```python
from build123d import *

# Parameters (mm, degrees)
SWEEP_THIN1_PROFILE_R    = 32
SWEEP_THIN1_PROFILE_R_2  = 22.5
SKETCH16_R               = 60
SKETCH16_R_2             = 7.5
SKETCH16_R_3             = 22.5
BOSS_EXTRUDE1_DEPTH      = 15
BOSS_EXTRUDE2_START      = 15
SKETCH17_R               = 60
SKETCH17_R_2             = 22.5
SKETCH17_R_3             = 7.5
BOSS_EXTRUDE2_DEPTH      = 15
SKETCH24_R               = 12
BOSS_EXTRUDE3_DEPTH      = 20
EXTRUDE_THIN1_REACH      = 577.336
EXTRUDE_THIN1_END_RADIUS = 32
SKETCH26_W               = 20
SKETCH26_H               = 64
RIB1_REACH               = 568.248
SKETCH27_WALL_W          = 1227.903575826
SKETCH27_WALL_H          = 24
SKETCH28_R               = 18
SKETCH28_R_2             = 12
BOSS_EXTRUDE4_DEPTH      = 8


with BuildPart() as part:
    # Sweep-Thin1: sweep along a path in Sketch1
    with BuildLine(Plane(origin=(0, 0, 0), x_dir=(0, 0, -1), z_dir=(1, 0, 0))) as sweep_thin1_path:
        Line((0, 0), (0, -135))
        ThreePointArc((0, -135), (-23.431457505, -191.568542495), (-80, -215))
        Line((-80, -215), (-445.82, -215))
    # Sweep-Thin1 profile (on start of the path) → Sweep-Thin1 (sweep)
    with BuildSketch(Plane(origin=(0, 0, 0), x_dir=(0, 0, -1), z_dir=(0, -1, 0))):
        Circle(SWEEP_THIN1_PROFILE_R)
        Circle(SWEEP_THIN1_PROFILE_R_2, mode=Mode.SUBTRACT)
    sweep(path=sweep_thin1_path.line)

    # Sketch16 → Boss-Extrude1 (add)
    with BuildSketch(Plane(origin=(0, 0, 0), x_dir=(1, 0, 0), z_dir=(0, 1, 0))):
        with Locations(Location((0, 0, 0), (0, 0, 270))):
            Circle(SKETCH16_R)
        with Locations(Location((0, -45, 0), (0, 0, 270))):
            Circle(SKETCH16_R_2, mode=Mode.SUBTRACT)
        with Locations(Location((-45, 0, 0), (0, 0, 270))):
            Circle(SKETCH16_R_2, mode=Mode.SUBTRACT)
        with Locations(Location((0, 45, 0), (0, 0, 270))):
            Circle(SKETCH16_R_2, mode=Mode.SUBTRACT)
        with Locations(Location((45, 0, 0), (0, 0, 270))):
            Circle(SKETCH16_R_2, mode=Mode.SUBTRACT)
        with Locations(Location((0, 0, 0), (0, 0, 90))):
            Circle(SKETCH16_R_3, mode=Mode.SUBTRACT)
    extrude(amount=BOSS_EXTRUDE1_DEPTH)

    # Sketch17 → Boss-Extrude2 (add)
    with BuildSketch(Plane.XY.offset(445.82).offset(BOSS_EXTRUDE2_START)):
        with Locations((0, -215)):
            Circle(SKETCH17_R)
        with Locations(Location((0, -215, 0), (0, 0, 270))):
            Circle(SKETCH17_R_2, mode=Mode.SUBTRACT)
        with Locations((0, -260)):
            Circle(SKETCH17_R_3, mode=Mode.SUBTRACT)
        with Locations((-45, -215)):
            Circle(SKETCH17_R_3, mode=Mode.SUBTRACT)
        with Locations((45, -215)):
            Circle(SKETCH17_R_3, mode=Mode.SUBTRACT)
        with Locations((0, -170)):
            Circle(SKETCH17_R_3, mode=Mode.SUBTRACT)
    extrude(amount=-BOSS_EXTRUDE2_DEPTH)



with BuildPart() as body_2:
    # Sketch24 → Boss-Extrude3 (new body)
    with BuildSketch(Plane(origin=(0, -325, 0), x_dir=(1, 0, 0), z_dir=(0, 1, 0))):
        with BuildLine():
            Line((15.39090645, -446.133712262), (97.89090645, -416.106167935))
            ThreePointArc((97.89090645, -416.106167935), (127.5, -373.82), (97.89090645, -331.533832065))
            Line((97.89090645, -331.533832065), (15.39090645, -301.506287738))
            ThreePointArc((15.39090645, -301.506287738), (0, -298.792455673), (-15.39090645, -301.506287738))
            Line((-15.39090645, -301.506287738), (-97.89090645, -331.533832065))
            ThreePointArc((-97.89090645, -331.533832065), (-127.5, -373.82), (-97.89090645, -416.106167935))
            Line((-97.89090645, -416.106167935), (-15.39090645, -446.133712262))
            ThreePointArc((-15.39090645, -446.133712262), (0, -448.847544327), (15.39090645, -446.133712262))
        make_face()
        with Locations(Location((-82.5, -373.82, 0), (0, 0, 270))):
            Circle(SKETCH24_R, mode=Mode.SUBTRACT)
        with Locations(Location((82.5, -373.82, 0), (0, 0, 270))):
            Circle(SKETCH24_R, mode=Mode.SUBTRACT)
    extrude(amount=BOSS_EXTRUDE3_DEPTH)


with BuildPart() as part_1:
    add(part.part)

    add(body_2.part)  # Extrude-Thin1 merges body 2
    # Extrude-Thin1: up to this cylinder (the profile starts outside it)
    extrude_thin1_end = Plane(origin=(0, -215, 373.82), z_dir=(0, 0, 1)) * Cylinder(EXTRUDE_THIN1_END_RADIUS, 1219.672, mode=Mode.PRIVATE)
    # Sketch26 → Extrude-Thin1 (add, up to the surface)
    with BuildSketch(Plane(origin=(0, -305, 0), x_dir=(1, 0, 0), z_dir=(0, 1, 0)), mode=Mode.PRIVATE) as extrude_thin1_sk1:
        with Locations((0, -373.82)):
            Rectangle(SKETCH26_W, SKETCH26_H)
    extrude_thin1_tool1 = extrude(extrude_thin1_sk1.sketch, amount=EXTRUDE_THIN1_REACH, mode=Mode.PRIVATE) - extrude_thin1_end
    add(extrude_thin1_tool1.solids().sort_by_distance((0, -305, 373.82))[0])

    # Sketch27 wall → Rib1 (add, up to next)
    with BuildSketch(Plane(origin=(44.5, -260, 385.82), x_dir=(-0.267643863786, 0.96351790963, 0), z_dir=(0.96351790963, 0.267643863786, 0)), mode=Mode.PRIVATE) as rib1_sk1:
        Rectangle(SKETCH27_WALL_W, SKETCH27_WALL_H)
    rib1_tool1 = extrude(rib1_sk1.sketch, amount=-RIB1_REACH, mode=Mode.PRIVATE) - part_1.part
    rib1 = rib1_tool1.solids().sort_by_distance((44.5, -260, 385.82))[0]
    add(rib1)

    # Mirror3: Rib1 across plane
    add(rib1.mirror(Plane(origin=(0, 0, 0), x_dir=(0, 0, 1), z_dir=(1, 0, 0))))

    # Sketch28 → Boss-Extrude4 (add)
    # profile 1 of 2: a face of its own
    with BuildSketch(Plane(origin=(0, -305, 0), x_dir=(1, 0, 0), z_dir=(0, 1, 0))):
        with Locations(Location((-82.5, -373.82, 0), (0, 0, 270))):
            Circle(SKETCH28_R)
        with Locations(Location((-82.5, -373.82, 0), (0, 0, 270))):
            Circle(SKETCH28_R_2, mode=Mode.SUBTRACT)
    # profile 2 of 2: a face of its own
    with BuildSketch(Plane(origin=(0, -305, 0), x_dir=(1, 0, 0), z_dir=(0, 1, 0))):
        with Locations(Location((82.5, -373.82, 0), (0, 0, 270))):
            Circle(SKETCH28_R)
        with Locations(Location((82.5, -373.82, 0), (0, 0, 270))):
            Circle(SKETCH28_R_2, mode=Mode.SUBTRACT)
    extrude(amount=BOSS_EXTRUDE4_DEPTH)


solid = part_1.part
```
Build history of the part. All positions in model axes, mm. A direction names the side the tool comes from. Give positions to 0.01 mm unless a question says otherwise; leave off trailing zeros. Order: outer loops, then holes, each group sorted by start corner. A loop starts at its lowest first (then second) coordinate and runs counter-clockwise, first axis right, second up. Notation, with made-up numbers: M 10,43 L 31,43 A23 cw 31,80 Z; hole C 88.5,21.25 d10. An arc over 180 degrees is marked long. Return JSON: item names as keys, results as strings.
Q1. Band-saw the part on A-A (z = 317). Give the cut face in (x, y).
Answer list:
{"outline": "M -57.96,-325 L 57.96,-325 L 57.96,-305 L -57.96,-305 Z; C 0,-215 d64; hole C 0,-215 d45"}
Q2. Flat gauge pins, fed straight in: pin 1 (5 mm diameter, centred on y = -240.5, z = 249, fed in from -X); pin 2 (24 mm diameter, centred on x = 0, z = 45, fed in from -Y); pin 3 (22 mm diameter, centred on x = 2.5, y = -274.5, fed in from -Z). Where does each tip first touch, or does it go through?
Answer list:
{"pin 1": "stops at x = -22.25", "pin 2": "stops at y = -244.61", "pin 3": "stops at z = 341.82"}
Q3. Wall check: probe 1 along Y at (x, z) = (0, 453); probe 2 along X at (y, z) = (-215, 220); probe 3 along Y at (x, z) = (-17.5, 399). Give the ranges that are in metal, low to high. Write a range as from..to.
Answer list:
{"probe 1": "y = -275..-267.5, -252.5..-237.5, -192.5..-177.5, -162.5..-155", "probe 2": "x = -32..-22.5, 22.5..32", "probe 3": "y = -325..-305, -241.79..-229.14, -200.86..-188.21"}
Q4. Two-plate mould, pull along X, no slides. Class faces 1 (the face through (-45.976, -207.564, 453.425)), 2 (the face through (37.68, 7.4, -1.63)), 3 (the face through (-26, 0, 26)), 4 (the face through (0.22, -315.14, 298.793)): pulls with the +X half, pulls with the -X half, needs draft (parallel to the pull), parting line crosses it, or undercut.
Answer list:
{"face 1": "undercut", "face 2": "undercut", "face 3": "needs draft", "face 4": "parting line crosses it"}
Q5. 3-axis set-ups, long thin cutter, end or side, ignore diameter. For faces 5 (the face through (-67.322, -301.056, 383.497)), 6 (the face through (31, -275, 373.82)), 7 (the face through (-31.24, -68.45, 6.94)), 8 (the face through (-0.976, -162.564, 453.425)), 9 (the face through (57.22, -315.14, 316.73)): which of +Z, -Z, +X, -X, +Y, -Y reach the whole face in a straight line?
Answer list:
{"face 5": "+Y", "face 6": "-Z", "face 7": "none", "face 8": "+Z", "face 9": "-Z, +X, -Y"}
Q6. Band-saw the part on B-B (x = 0). Count the separate pieces of the cut face and the enclosed holes in it, then the cut area to 3 significant figures.
Answer list:
{"separate pieces": "6", "enclosed holes": "0", "area": "20,000 mm^2"}
Q7. Band-saw the part on C-C (x = 45). Give the cut face in (y, z), then the cut area to 3 significant figures.
Answer list:
{"outline": "M -325,312.28 L -305,312.28 L -305,373.82 L -261.8,373.82 L -261.8,397.82 L -305,397.82 L -305,435.36 L -325,435.36 Z; M -254.69,445.82 L -222.5,445.82 L -222.5,460.82 L -254.69,460.82 Z; M -207.5,445.82 L -175.31,445.82 L -175.31,460.82 L -207.5,460.82 Z; M 0,-39.69 L 15,-39.69 L 15,-7.5 L 0,-7.5 Z; M 0,7.5 L 15,7.5 L 15,39.69 L 0,39.69 Z", "area": "5,430 mm^2"}
Q8. Band-saw the part on D-D (z = 214.5). Give the cut face in (x, y).
Answer list:
{"outline": "C 0,-215 d64; hole C 0,-215 d45"}
